Design review of the part built by this model. Coordinates are the model's own, in mm. Face numbers are marked on the shaded views. A direction names the side the tool comes from. Round coordinates to 2 decimals unless told otherwise and drop trailing zeros. Order: outer loops, then holes, each group sorted by start corner. A loop starts at its lowest first (then second) coordinate and runs counter-clockwise, first axis right, second up. Notation, with made-up numbers: (-26, -1.5) - (-2, -1.5) arc R26 cw to (-2, 22.5) - close; hole circle Ø1 at (79, -4). An arc over 180 degrees is marked (long way). Use CSV: the item, a comma, the result in double quotes.
from build123d import *

# Parameters (mm, degrees)
SKETCH1_W           = 12.7
SKETCH1_H           = 12.7
BOSS_EXTRUDE1_DEPTH = 2.54
FILLET1_R           = 0.635
SHELL1_START        = 0.635
SHELL1_OUTLINE_W    = 1.905
SHELL1_OUTLINE_H    = 11.43
SHELL1_DEPTH        = 11.43
SKETCH2_R           = 2.54
BOSS_EXTRUDE2_DEPTH = 1.905
BOSS_EXTRUDE4_DEPTH = 0.00254


# Read off the part's stored shape, not the designer's step: Shell1
with BuildPart() as part:
    # Sketch1 → Boss-Extrude1 (new body)
    with BuildSketch(Plane(origin=(0, 0, 0), x_dir=(1, 0, 0), z_dir=(0, 1, 0))):
        with Locations((6.35, 6.35)):
            Rectangle(SKETCH1_W, SKETCH1_H)
    extrude(amount=BOSS_EXTRUDE1_DEPTH)

    # Fillet1
    fillet1_edges = [part.edges().sort_by_distance(p)[0] for p in [
        (0, 1.27, -12.7),
        (12.7, 1.27, -12.7),
        (12.7, 1.27, 0),
        (0, 1.27, 0),
    ]]
    fillet(fillet1_edges, radius=FILLET1_R)

    # Shell1 outline → Shell1 (cut)
    with BuildSketch(Plane.YZ.offset(SHELL1_START)):
        with Locations((0.9525, -6.35)):
            Rectangle(SHELL1_OUTLINE_W, SHELL1_OUTLINE_H)
    extrude(amount=SHELL1_DEPTH, mode=Mode.SUBTRACT)

    # Sketch2 → Boss-Extrude2 (add)
    with BuildSketch(Plane(origin=(0, 1.905, 0), x_dir=(-1, 0, 0), z_dir=(0, -1, 0))):
        with Locations(Location((-6.35, 6.35, 0), (0, 0, 270))):
            Circle(SKETCH2_R)
    extrude(amount=BOSS_EXTRUDE2_DEPTH)

    # Sketch4 → Boss-Extrude4 (add)
    with BuildSketch(Plane(origin=(0, 2.54, 0), x_dir=(1, 0, 0), z_dir=(0, 1, 0))):
        Polygon((6.040641026, 5.796410256), (6.976858974, 5.796410256), (6.976858974, 5.26724359), (6.610512821, 5.26724359), (6.610512821, 2.214358974), (6.976858974, 2.214358974), (6.976858974, 1.685192308), (6.040641026, 1.685192308), align=None)
        with BuildLine():
            Line((5.501705128, 8.769512821), (5.501705128, 9.298679487))
            add(Edge.make_bspline(
                [(5.501705128, 9.298679487), (5.532724551, 9.300577954), (5.590656774, 9.304123553), (5.670981575, 9.318580211), (5.738741024, 9.339627117), (5.795240216, 9.368692195), (5.841347316, 9.407649179), (5.880872771, 9.454311284), (5.914137334, 9.51039725), (5.937186765, 9.563561565), (5.953049789, 9.612405831), (5.963005648, 9.655837142), (5.971085115, 9.705154512), (5.97787015, 9.760121424), (5.983848589, 9.821176644), (5.987184914, 9.888028776), (5.990050912, 9.960961441), (5.990127023, 10.011439709), (5.990166667, 10.037731971)],
                knots=[0, 0, 0, 0, 1.451517752, 2.710870899, 3.804446884, 4.757414975, 5.658161607, 6.607155001, 7.602945962, 8.694545061, 9.30871163, 10.000889012, 10.774639975, 11.643541707, 12.589063004, 13.641044214, 14.771307238, 16, 16, 16, 16], degree=3))
            add(Edge.make_bspline(
                [(5.990166667, 10.037731971), (5.99027291, 10.070806168), (5.990475881, 10.133992465), (5.992430984, 10.224740262), (5.995391945, 10.307239275), (6.000125578, 10.381629312), (6.004576412, 10.448111322), (6.011928876, 10.506142904), (6.018937818, 10.556415186), (6.031654225, 10.611230568), (6.050499963, 10.67120317), (6.079363112, 10.735660672), (6.113646688, 10.792741786), (6.154613928, 10.843272465), (6.204455745, 10.88728976), (6.263366728, 10.926601221), (6.332418843, 10.96169463), (6.396939353, 10.986683085), (6.454324586, 11.005661541), (6.50346794, 11.016391589), (6.556837627, 11.026835102), (6.61501627, 11.034947693), (6.677817883, 11.041279814), (6.745295804, 11.045379799), (6.817163158, 11.049034753), (6.866593581, 11.04901181), (6.892039663, 11.049)],
                knots=[0, 0, 0, 0, 1.46534077, 2.799446828, 4.021441889, 5.122390044, 6.102149716, 6.972462297, 7.7137374, 8.349485774, 9.463459583, 10.49348432, 11.471305969, 12.40580496, 13.363708508, 14.405783216, 15.535837735, 16.788212615, 17.468477195, 18.211238595, 19.014437677, 19.877880266, 20.812520865, 21.810349341, 22.872798814, 24, 24, 24, 24], degree=3))
            Line((6.892039663, 11.049), (7.007794872, 11.049))
            Line((7.007794872, 11.049), (7.007794872, 10.519833333))
            add(Edge.make_bspline(
                [(7.007794872, 10.519833333), (6.989139417, 10.519587027), (6.953312265, 10.519114005), (6.902192532, 10.51898063), (6.856196849, 10.516761047), (6.815211942, 10.514648161), (6.779444801, 10.510463786), (6.748361679, 10.507065532), (6.722625011, 10.502147344), (6.69568576, 10.49451003), (6.667022453, 10.483581701), (6.637681703, 10.465672367), (6.612925486, 10.444240108), (6.591660898, 10.418455284), (6.577004821, 10.383512508), (6.566766404, 10.339311488), (6.560706101, 10.283818342), (6.560274859, 10.243181314), (6.560038462, 10.220905048)],
                knots=[0, 0, 0, 0, 1.386539278, 2.662800514, 3.798152769, 4.808447339, 5.711450255, 6.473580847, 7.131722202, 7.655446357, 8.553625873, 9.402064563, 10.195002251, 10.979916755, 11.86135854, 12.980969535, 14.34503827, 16, 16, 16, 16], degree=3))
            add(Edge.make_bspline(
                [(6.560038462, 10.220905048), (6.559545706, 10.176381457), (6.558534177, 10.084983372), (6.554177156, 9.943947845), (6.545761586, 9.795526586), (6.537956266, 9.694057712), (6.533961739, 9.642129006)],
                knots=[0, 0, 0, 0, 0.92200247, 1.892687869, 2.921541302, 4, 4, 4, 4], degree=3))
            add(Edge.make_bspline(
                [(6.533961739, 9.642129006), (6.530117819, 9.608277323), (6.522539172, 9.541535565), (6.497126743, 9.445069771), (6.461748345, 9.353690497), (6.429734003, 9.297479672), (6.413754407, 9.269422676)],
                knots=[0, 0, 0, 0, 1.03352617, 2.037693405, 3.020536894, 4, 4, 4, 4], degree=3))
            add(Edge.make_bspline(
                [(6.413754407, 9.269422676), (6.399275564, 9.248804803), (6.368653828, 9.205199448), (6.307860152, 9.146179587), (6.235183983, 9.086222662), (6.179303029, 9.050855916), (6.149807091, 9.032188101)],
                knots=[0, 0, 0, 0, 0.843495541, 1.78393383, 2.830282145, 4, 4, 4, 4], degree=3))
            add(Edge.make_bspline(
                [(6.149807091, 9.032188101), (6.173049633, 9.016766999), (6.218724746, 8.986462199), (6.280720945, 8.933109752), (6.333920011, 8.872989352), (6.380789418, 8.807176718), (6.419813309, 8.733359395), (6.452416847, 8.6512131), (6.476240614, 8.55922335), (6.486596694, 8.49464301), (6.491984575, 8.461044271)],
                knots=[0, 0, 0, 0, 0.968830733, 1.903899033, 2.832763283, 3.752700456, 4.705369692, 5.727457187, 6.817680861, 8, 8, 8, 8], degree=3))
            add(Edge.make_bspline(
                [(6.491984575, 8.461044271), (6.493146133, 8.451300636), (6.495967556, 8.427633362), (6.497777051, 8.385555815), (6.50116022, 8.330878989), (6.505264993, 8.263278599), (6.507854941, 8.182882253), (6.512052118, 8.089623889), (6.515713081, 7.98361332), (6.518082021, 7.908557532), (6.519333333, 7.868911859)],
                knots=[0, 0, 0, 0, 0.397118983, 0.964601375, 1.703940229, 2.615138326, 3.70595647, 4.960054814, 6.394252129, 8, 8, 8, 8], degree=3))
            add(Edge.make_bspline(
                [(6.519333333, 7.868911859), (6.520579054, 7.841114333), (6.522806566, 7.791408715), (6.528797656, 7.725746662), (6.534024869, 7.676794658), (6.54216353, 7.65090783), (6.545410056, 7.64058153)],
                knots=[0, 0, 0, 0, 1.448250494, 2.589661623, 3.437413606, 4, 4, 4, 4], degree=3))
            add(Edge.make_bspline(
                [(6.545410056, 7.64058153), (6.551354746, 7.630113272), (6.56339075, 7.608918561), (6.589875696, 7.581725399), (6.622903191, 7.55908913), (6.655245791, 7.542548203), (6.686799456, 7.533078155), (6.716248693, 7.52590647), (6.751399708, 7.520618856), (6.7918716, 7.515397976), (6.837928889, 7.51173648), (6.88946915, 7.509224277), (6.946733128, 7.508161361), (6.986806182, 7.507828294), (7.007794872, 7.507653846)],
                knots=[0, 0, 0, 0, 0.854656799, 1.730393381, 2.672957062, 3.699349592, 4.301036757, 5.015168751, 5.856653451, 6.830503664, 7.921393134, 9.14589491, 10.505131993, 12, 12, 12, 12], degree=3))
            Line((7.007794872, 7.507653846), (7.007794872, 6.978487179))
            Line((7.007794872, 6.978487179), (6.892039663, 6.978487179))
            add(Edge.make_bspline(
                [(6.892039663, 6.978487179), (6.866383077, 6.978526215), (6.816963917, 6.978601404), (6.745307814, 6.981504501), (6.678867696, 6.984758361), (6.61746922, 6.991144216), (6.561045697, 6.996538747), (6.50982297, 7.005993345), (6.463681374, 7.015763286), (6.409658587, 7.030867229), (6.349044044, 7.054494053), (6.282121034, 7.08767088), (6.223475812, 7.128634915), (6.170084284, 7.173473086), (6.125792724, 7.226665597), (6.086748214, 7.284923434), (6.056128199, 7.350373385), (6.035010547, 7.409747118), (6.021564816, 7.462998966), (6.01394496, 7.510317213), (6.005784949, 7.563862295), (6.000793847, 7.624440305), (5.995228131, 7.691595022), (5.992493569, 7.765435518), (5.990466407, 7.845791113), (5.990269319, 7.901558967), (5.990166667, 7.930605569)],
                knots=[0, 0, 0, 0, 1.180076656, 2.27303809, 3.298707054, 4.239039526, 5.112461827, 5.904507711, 6.633329935, 7.281697308, 8.48250633, 9.620862782, 10.708284457, 11.766090354, 12.817538401, 13.88054636, 14.984116166, 16.131501886, 16.774862487, 17.507589143, 18.335104889, 19.265728017, 20.302418806, 21.434743744, 22.663890185, 24, 24, 24, 24], degree=3))
            add(Edge.make_bspline(
                [(5.990166667, 7.930605569), (5.990037977, 7.963042723), (5.989792348, 8.02495516), (5.988132762, 8.113818002), (5.98420043, 8.194387809), (5.979333537, 8.266723087), (5.972920121, 8.330771786), (5.965735187, 8.386687047), (5.95627693, 8.434472879), (5.942293856, 8.486214809), (5.920195452, 8.541572567), (5.888317363, 8.600377736), (5.848148398, 8.649211105), (5.801607935, 8.690417629), (5.744582017, 8.723334024), (5.67496369, 8.746517187), (5.592703317, 8.763035254), (5.533381357, 8.767257997), (5.501705128, 8.769512821)],
                knots=[0, 0, 0, 0, 1.386030809, 2.645501613, 3.797256415, 4.832502903, 5.742904192, 6.547458989, 7.240326361, 7.822704252, 8.835390849, 9.780379381, 10.668884048, 11.522772015, 12.423932252, 13.461079439, 14.644289055, 16, 16, 16, 16], degree=3))
        make_face()
    extrude(amount=BOSS_EXTRUDE4_DEPTH)


solid = part.part
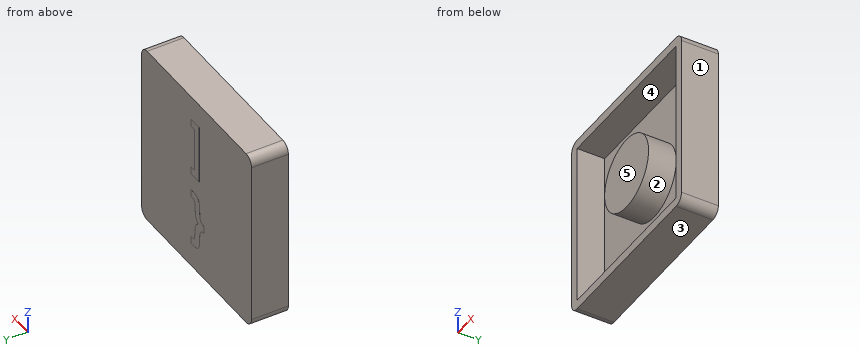
1) For the marked faces 1 and 2, list the 3-axis set-ups (+Z, -Z, +X, -X, +Y, -Y) from which the entire face can be reached by the end or side of a thin tool; tool diameter is ignored.
Data:
face 1,"+Z, -Z, +X, +Y, -Y"
face 2,"-Y"
2) Insertion check: pin 1 Ø4 at (x, z) = (9.5, -10.5) entering from +Y; pin 2 Ø2 at (x, z) = (8.5, -10.5) entering from -Y (3 decimals). Each pin has a flat end and moves straight along its axis. Give the tip position at first contact, or say it passes through.
Data:
pin 1,"stops at y = 2.54"
pin 2,"stops at y = 1.905"
3) To check wall thickness, follow L1, parallel to Z at x = 2, y = 1 (3 decimals); L2, parallel to Z at x = 6.25, y = 1.3 (3 decimals); L3, parallel to X at y = 0.6, z = -2 (3 decimals). State the ranges of each line that lie inside material, in increasing order. Write a range as from..to.
Data:
L1,"z = -12.7..-12.065, -0.635..0"
L2,"z = -12.7..-12.065, -8.888..-3.812, -0.635..0"
L3,"x = 0..0.635, 12.065..12.7"
4) The part is to be moulded in two halves that separate along Z. For the marked faces 3, 4 and 5, say which applies: +Z half, -Z half, draft (parallel to the pull), parting line (faces both ways), or undercut.
Data:
face 3,"-Z half"
face 4,"undercut"
face 5,"draft"
5) We need section C-C (x = 1.25). Give the boundary of the cut face in (y, z) (3 decimals).
Data:
outline,"(0, -12.7) - (2.54, -12.7) - (2.54, 0) - (0, 0) - (0, -0.635) - (1.905, -0.635) - (1.905, -12.065) - (0, -12.065) - close"
6) We need section A-A (y = 1.3). Give the boundary of the cut face in (x, z) (3 decimals).
Data:
outline,"(0, -12.065) arc R0.635 ccw to (0.635, -12.7) - (12.065, -12.7) arc R0.635 ccw to (12.7, -12.065) - (12.7, -0.635) arc R0.635 ccw to (12.065, 0) - (0.635, 0) arc R0.635 ccw to (0, -0.635) - close; circle Ø5.08 at (6.35, -6.35); hole (0.635, -12.065) - (12.065, -12.065) - (12.065, -0.635) - (0.635, -0.635) - close"
